Input: part model. Units: mm. Frame: model coordinates. Give positions to 0.01 mm unless a question says otherwise; leave off trailing zeros. Write each loop counter-clockwise with the first axis right and the second up, starting at its lowest first coordinate (ties: lowest second). Pieces come first, ordered by that corner, then holes. Notation, with made-up numbers: (46, 6.25) -> (86, 6.25) arc R11 ccw to (86, 20.25) -> close; hole circle Ø4 at (14.25, 27.25). An arc over 180 degrees is marked (long way). Return JSON: item names as keys, results as strings. Group by question number.
Item 1: Section A-A, the plane z = -12.7. Return loops of the section in (x, y).
Item 2: Pin query (flat end, axial travel): P1, Ø6.5, axis at x = 12.7, z = -88.9, coming from the +Y side; P2, Ø0.8, axis at y = 1, z = -54, coming from the +X side; P3, Ø0.8, axis at y = 1, z = -139, coming from the +X side. Return the tip coordinate at first contact, or that it passes through.
Item 3: Section B-B, the plane x = 88.9. Return loops of the section in (y, z).
Item 4: Section C-C, the plane x = 12.7. Count the separate pieces of the cut face and the enclosed holes in it, then the cut area to 3 significant figures.
Item 5: Line query: line 1 (X direction, y = 0.7, z = -88.9); line 2 (X direction, y = 1.05, z = -63.5); line 3 (X direction, y = 1.25, z = -138.5). Output: solid intervals per line, ascending. Write a range as [from, to].
from build123d import *

# Parameters (mm, degrees)
BOSS_EXTRUDE1_DEPTH        = 1.5875
F_9_0_196_DIAMETER_HOLE1_D = 4.9784
LPATTERN1_COUNT            = 4
LPATTERN1_PITCH            = 25.4
LPATTERN1_COL_COUNT        = 4
LPATTERN1_COL_PITCH        = 25.4
LPATTERN2_COUNT            = 4
LPATTERN2_PITCH            = 25.4
FILLET1_R                  = 3.175


with BuildPart() as part:
    # Sketch1 → Boss-Extrude1 (new body)
    with BuildSketch(Plane(origin=(0, 0, 0), x_dir=(1, 0, 0), z_dir=(0, 1, 0))):
        Polygon((101.6, 101.6), (101.6, 76.2), (25.4, 0), (0, 0), (0, 177.8), (25.4, 177.8), align=None)
        Polygon((25.4, 17.960512242), (83.639487758, 76.2), (25.4, 76.2), align=None, mode=Mode.SUBTRACT)
        Polygon((83.639487758, 101.6), (25.4, 159.839487758), (25.4, 101.6), align=None, mode=Mode.SUBTRACT)
    extrude(amount=BOSS_EXTRUDE1_DEPTH)

    # #9 (0.196) Diameter Hole1 (through all)
    with Locations(Plane(origin=(12.7, 1.5875, -88.9), x_dir=(0, 0, 1), z_dir=(0, 1, 0))):
        with Locations((0, 0)):
            f_9_0_196_diameter_hole1 = Hole(F_9_0_196_DIAMETER_HOLE1_D / 2)

    # LPattern1: #9 (0.196) Diameter Hole1 ×4
    with Locations(*[(0, 0, -i * LPATTERN1_PITCH) for i in range(1, LPATTERN1_COUNT)]):
        add(f_9_0_196_diameter_hole1, mode=Mode.SUBTRACT)

    # LPattern1 col: #9 (0.196) Diameter Hole1 ×4
    with Locations(*[(i * LPATTERN1_COL_PITCH, 0, 0) for i in range(1, LPATTERN1_COL_COUNT)]):
        add(f_9_0_196_diameter_hole1, mode=Mode.SUBTRACT)

    # LPattern2: #9 (0.196) Diameter Hole1 ×4
    with Locations(*[(0, 0, i * LPATTERN2_PITCH) for i in range(1, LPATTERN2_COUNT)]):
        add(f_9_0_196_diameter_hole1, mode=Mode.SUBTRACT)

    # Fillet1
    fillet1_edges = [part.edges().sort_by_distance(p)[0] for p in [
        (101.6, 0.79375, -76.2),
        (25.4, 0.79375, 0),
        (0, 0.79375, 0),
        (0, 0.79375, -177.8),
        (25.4, 0.79375, -177.8),
        (101.6, 0.79375, -101.6),
        (25.4, 0.79375, -159.839487758),
        (25.4, 0.79375, -101.6),
        (83.639487758, 0.79375, -101.6),
        (83.639487758, 0.79375, -76.2),
        (25.4, 0.79375, -76.2),
        (25.4, 0.79375, -17.960512242),
    ]]
    fillet(fillet1_edges, radius=FILLET1_R)


solid = part.part
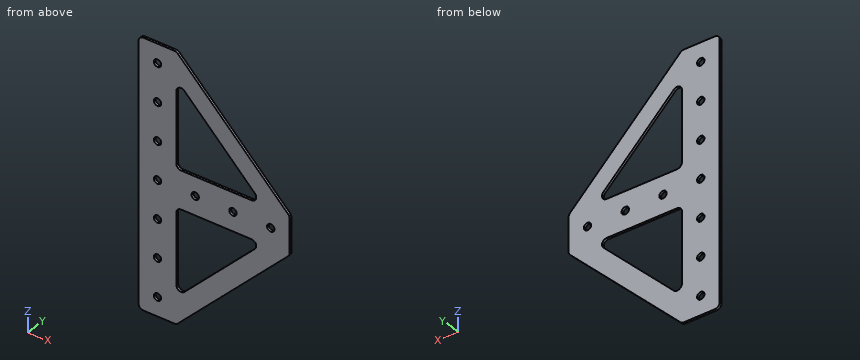
Answer below:
{
 "1": {"outline": "(0, 0) -> (10.21, 0) -> (10.21, 1.59) -> (0, 1.59) -> close; (15.19, 0) -> (38.1, 0) -> (38.1, 1.59) -> (15.19, 1.59) -> close"},
 "2": {"P1": "stops at y = 1.59", "P2": "stops at x = 79.8", "P3": "stops at x = 64.6"},
 "3": {"outline": "(0, -114.3) -> (1.59, -114.3) -> (1.59, -91.39) -> (0, -91.39) -> close; (0, -86.41) -> (1.59, -86.41) -> (1.59, -63.5) -> (0, -63.5) -> close"},
 "4": {"separate pieces": "8", "enclosed holes": "0", "area": "227 mm2"},
 "5": {"line 1": "x = [0, 10.21], [15.19, 35.61], [40.59, 61.01], [65.99, 86.41], [91.39, 101.6]", "line 2": "x = [0, 10.21], [15.19, 25.4], [70.94, 88.9]", "line 3": "x = [0, 10.52], [14.88, 25.4], [46.74, 64.7]"}
}
